Here's how the part is built. I have some questions about the finished solid (model axes, mm). A direction names the side the tool comes from. Round coordinates to 2 decimals unless told otherwise and drop trailing zeros. Order: outer loops, then holes, each group sorted by start corner. A loop starts at its lowest first (then second) coordinate and runs counter-clockwise, first axis right, second up. Notation, with made-up numbers: (41.25, -21.5) -> (54.25, -21.5) arc R21 cw to (54.25, 7.5) -> close; hole circle Ø8 at (15, -32.5). An arc over 180 degrees is marked (long way). Use a Markdown table: item, result. Add a question column.
(1) I want a section at C-C, the plane x = 10. Please give me the cut outline in (y, z), then the cut area to 3 significant figures.
(2) I want a section at B-B, the plane y = -3.25. Please give me the cut outline in (x, z).
(3) I want a section at D-D, the plane x = 4.25. Please give me the cut outline in (y, z).
(4) I'm going to push flat-ended pins straight in: P1, Ø5, axis at x = 8.5, z = 1.5, coming from the +Y side; P2, Ø3, axis at x = 12, y = 1, coming from the -Z side; P3, Ø3, axis at x = 7.5, z = 2, coming from the -Y side. Where does each tip first touch, or does it pass through?
(5) If I drill on probe 1 along Y at (x, z) = (3.7, -15); probe 2 along Z at (x, y) = (4, 0.5), over which ranges is the centre line in solid material (lowest first)?
(6) On a 3-axis mill with a long thin cutter (end or side, diameter ignored), from which of +Z, -Z, +X, -X, +Y, -Y can I reach the whole of each face in a straight line? I mean faces 1 (the face through (12.2, -5, -0.1)), 2 (the face through (12.2, 5, 0.1)), 3 (the face through (10, 0, -10)), 4 (the face through (10, 0, 10)). Say none if no direction works.
(7) Thinking about a two-plate mould opening in X: for faces 5 (the face through (8.4, 0.1, 1.2)), 6 (the face through (2, 10, 0)), 7 (the face through (15, 0, 0)), 8 (the face through (0, 0, 0)), which applies, pulls with the +X half, pulls with the -X half, needs draft (parallel to the pull), parting line crosses it, or undercut?
(8) I want a section at A-A, the plane z = 0. Please give me the cut outline in (x, y), then the cut area to 3 significant figures.
Autodesk Inventor part; units mm, degrees
ref_plane "YZ Plane" through (0, 0, 0) normal (1, 0, 0) x (0, 1, 0)
ref_plane "XZ Plane" through (0, 0, 0) normal (0, 1, 0) x (-1, 0, 0)
ref_plane "XY Plane" through (0, 0, 0) normal (0, 0, 1) x (1, 0, 0)
sketch "草图1" plane through (0, 0, 0) normal (1, 0, 0) x (0, 1, 0)
  line L0 (10, 20) -> (-10, 20)
  line L1 (-10, 20) -> (-10, -20)
  line L2 (-10, -20) -> (10, -20)
  line L3 (10, -20) -> (10, 20)
  point P0 (0, 0)
  dimension "d0" = 20
  dimension "d1" = 40
extrude "拉伸1" add sketch "草图1" along normal blind 5
sketch "草图2" plane through (5, 0, 0) normal (1, 0, 0) x (0, 0, -1)
  circle A0 centre (-15, 0) radius 2
  point P0 (0, 0)
  dimension "d4" = 4
extrude "拉伸2" cut sketch "草图2" against normal through all
sketch "草图3" plane through (5, 0, 0) normal (1, 0, 0) x (0, 0, -1)
  circle A0 centre (15, 0) radius 2
  point P0 (0, 0)
  dimension "d7" = 4
extrude "拉伸3" cut sketch "草图3" against normal through all
sketch "草图4" plane through (5, 0, 0) normal (1, 0, 0) x (0, 0, -1)
  line L0 (-10, 5) -> (10, 5)
  line L1 (10, 5) -> (10, -5)
  line L2 (10, -5) -> (-10, -5)
  line L3 (-10, -5) -> (-10, 5)
  point P0 (0, 0)
  dimension "d10" = 20
  dimension "d11" = 10
extrude "拉伸4" add sketch "草图4" along normal blind 10
sketch "草图5" plane through (5, 5, 10) normal (0, 1, 0) x (1, 0, 0)
  circle A0 centre (5, 10) radius 2
  point P0 (-5, 10)
  dimension "d14" = 4
extrude "拉伸5" cut sketch "草图5" against normal through all
sketch "草图6" plane through (5, 0, 0) normal (1, 0, 0) x (0, 0, -1)
  point P0 (0, 0)
equation "\"折弯半径\" = 厚度"
equation "\"折弯释压宽度\" = 厚度"
equation "\"折弯释压深度\" = 0.5 * 厚度"
equation "\"拐角释压尺寸\" = 4 * 厚度"
equation "\"最小余量\" = 2 * 厚度"
equation "\"过渡半径\" = 折弯半径"
equation "\"Jacobi半径尺寸\" = 折弯半径"
equation "\"间隙大小\" = 厚度"
properties part number "滑竿固定器"
Taken from the geometry:
| question | item | result |
|---|---|---|
| 1 | outline | (-5, -10) -> (5, -10) -> (5, -2) -> (-5, -2) -> close; (-5, 2) -> (5, 2) -> (5, 10) -> (-5, 10) -> close |
| 1 | area | 160 mm2 |
| 2 | outline | (0, -20) -> (5, -20) -> (5, -10) -> (15, -10) -> (15, 10) -> (5, 10) -> (5, 20) -> (0, 20) -> close; hole circle Ø4 at (10, 0) |
| 3 | outline | (-10, -20) -> (10, -20) -> (10, 20) -> (-10, 20) -> close; hole circle Ø4 at (0, -15); hole circle Ø4 at (0, 15) |
| 4 | P1 | stops at y = 5 |
| 4 | P2 | stops at z = -10 |
| 4 | P3 | stops at y = -5 |
| 5 | probe 1 | y = -10 to -2, 2 to 10 |
| 5 | probe 2 | z = -20 to -16.94, -13.06 to 13.06, 16.94 to 20 |
| 6 | face 1 | +Z, -Z, +X, -Y |
| 6 | face 2 | +Z, -Z, +X, +Y |
| 6 | face 3 | -Z, +X, +Y, -Y |
| 6 | face 4 | +Z, +X, +Y, -Y |
| 7 | face 5 | undercut |
| 7 | face 6 | needs draft |
| 7 | face 7 | pulls with the +X half |
| 7 | face 8 | pulls with the -X half |
| 8 | outline | (0, -10) -> (5, -10) -> (5, -5) -> (8, -5) -> (8, 5) -> (5, 5) -> (5, 10) -> (0, 10) -> close; (12, -5) -> (15, -5) -> (15, 5) -> (12, 5) -> close |
| 8 | area | 160 mm2 |
